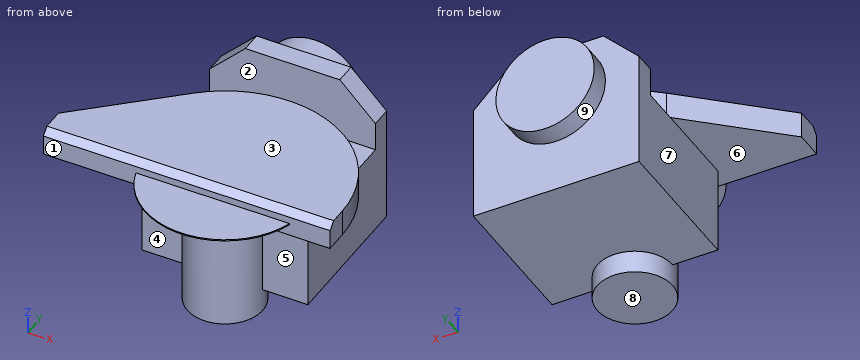
from build123d import *

# Parameters (mm, degrees)
SKETCH1_R                = 225
BOSS_EXTRUDE1_DEPTH      = 3.5
SKETCH2_R                = 105.863842181
BOSS_EXTRUDE2_DEPTH      = 350
SKETCH3_W                = 465.371554394
SKETCH3_H                = 246.036459022
BOSS_EXTRUDE3_DEPTH      = 350
BOSS_EXTRUDE4_DEPTH      = 38
BOSS_EXTRUDE4_DEPTH_BACK = 36
CUT_EXTRUDE1_DEPTH       = 1011
BOSS_EXTRUDE5_DEPTH      = 58
SKETCH7_R                = 138.083103167
BOSS_EXTRUDE6_DEPTH      = 58


with BuildPart() as part:
    # Sketch1 → Boss-Extrude1 (new body)
    with BuildSketch(Plane.XY):
        Circle(SKETCH1_R)
    extrude(amount=BOSS_EXTRUDE1_DEPTH)

    # Sketch2 → Boss-Extrude2 (add)
    with BuildSketch(Plane(origin=(0, 0, 0), x_dir=(-1, 0, 0), z_dir=(0, 0, -1))):
        Circle(SKETCH2_R)
    extrude(amount=BOSS_EXTRUDE2_DEPTH)

    # Sketch3 → Boss-Extrude3 (add)
    with BuildSketch(Plane(origin=(0, 0, 0), x_dir=(1, 0, 0), z_dir=(0, 1, 0))):
        with Locations((0, 162.855088027)):
            Rectangle(SKETCH3_W, SKETCH3_H)
    extrude(amount=BOSS_EXTRUDE3_DEPTH)

    # Sketch4 → Boss-Extrude4 (add, two sides: drawn at the far end of the back side and taken through both)
    with BuildSketch(Plane.XY.offset(3.5).offset(-BOSS_EXTRUDE4_DEPTH_BACK)):
        with BuildLine():
            Line((-475.524623773, -63.931124179), (329.566599898, -63.931124179))
            Line((329.566599898, -63.931124179), (329.566599898, 0))
            ThreePointArc((329.566599898, 0), (133.661871779, 301.245162287), (-221.148477595, 244.351170707))
            Line((-221.148477595, 244.351170707), (-475.524623773, 14.129652631))
            Line((-475.524623773, 14.129652631), (-475.524623773, -63.931124179))
        make_face()
    extrude(amount=BOSS_EXTRUDE4_DEPTH + BOSS_EXTRUDE4_DEPTH_BACK)

    # Sketch5 → Cut-Extrude1 (cut)
    with BuildSketch(Plane(origin=(329.566599898, 0, 0), x_dir=(0, 0, -1), z_dir=(1, 0, 0))):
        Polygon((-41.5, -63.931124179), (-41.5, -45.396753324), (-22.965629146, -63.931124179), align=None)
    extrude(amount=-CUT_EXTRUDE1_DEPTH, mode=Mode.SUBTRACT)

    # Sketch6 → Boss-Extrude5 (add)
    with BuildSketch(Plane(origin=(0, 350, 0), x_dir=(1, 0, 0), z_dir=(0, 1, 0))):
        Polygon((-232.685777197, 285.873317538), (232.685777197, 285.873317538), (232.685777197, -41.230401705), (132.685777197, -141.230401705), (-132.685777197, -141.230401705), (-232.685777197, -41.230401705), align=None)
    extrude(amount=BOSS_EXTRUDE5_DEPTH)

    # Sketch7 → Boss-Extrude6 (add)
    with BuildSketch(Plane(origin=(0, 408, 0), x_dir=(1, 0, 0), z_dir=(0, 1, 0))):
        with Locations(Location((0, 0, 0), (0, 0, 270))):
            Circle(SKETCH7_R)
    extrude(amount=BOSS_EXTRUDE6_DEPTH)


solid = part.part
Can you work these out from the model? Positions are in its coordinate system, mm. Face numbers are marked on the shaded views. A direction names the side the tool comes from. Give positions to 0.01 mm unless a question says otherwise; leave off trailing zeros. Loops run counter-clockwise (first coordinate to the right, second up) from the corner with the lowest first, then second, coordinate; pieces in that order, holes last. Notation, with made-up numbers: (51, -12) - (99, -12) arc R16 cw to (99, 17) - close; hole circle Ø1 at (-34, -14). An arc over 180 degrees is marked (long way). Return JSON: item names as keys, results as strings.
1. For the marked faces 1, 2, 3, 4 and 5, which set-ups out of +Z, -Z, +X, -X, +Y, -Y let a thin tool reach every point of the face, with its end or its side?
Output values:
{"face 1": "-Y", "face 2": "+Z, +X, -X", "face 3": "+Z, +X, -X, -Y", "face 4": "-Z, -X, -Y", "face 5": "-Z, +X, -Y"}
2. I want a section at B-B on z = -275. Please give me the cut outline in (x, y), and give its area (3 significant figures).
Output values:
{"outline": "(-232.69, 0) - (-105.86, 0) arc R105.86 ccw to (105.86, 0) - (232.69, 0) - (232.69, 408) - (-232.69, 408) - close", "area": "207,000 mm²"}
3. I want a section at A-A on x = 0. Please give me the cut outline in (y, z), and give its area (3 significant figures).
Output values:
{"outline": "(-225, 0) - (-105.86, 0) - (-105.86, -350) - (105.86, -350) - (105.86, -285.87) - (408, -285.87) - (408, -138.08) - (466, -138.08) - (466, 138.08) - (408, 138.08) - (408, 141.23) - (350, 141.23) - (350, -39.84) - (105.86, -39.84) - (105.86, -32.5) - (329.57, -32.5) - (329.57, 41.5) - (-45.4, 41.5) - (-63.93, 22.97) - (-63.93, 3.5) - (-225, 3.5) - close", "area": "199,000 mm²"}
4. If I drill on line 1 (Z direction, x = -71, y = 213); line 2 (Z direction, x = -103.5, y = -157); line 3 (Y direction, x = 98, z = -139), over which ranges is the centre line in solid material (lowest first)?
Output values:
{"line 1": "z = -285.87 to -39.84, -32.5 to 41.5", "line 2": "z = 0 to 3.5", "line 3": "y = -40.04 to 408"}
5. I want a section at C-C on y = 133.5. Please give me the cut outline in (x, z).
Output values:
{"outline": "(-343.63, -32.5) - (301.32, -32.5) - (301.32, 41.5) - (-343.63, 41.5) - close; (-232.69, -285.87) - (232.69, -285.87) - (232.69, -39.84) - (-232.69, -39.84) - close"}
6. I'm going to push flat-ended pins straight in: pin 1 Ø1.5 at (x, y) = (175.5, -118.5) entering from +Z; pin 2 Ø3 at (x, y) = (-12, 346) entering from +Z; pin 3 Ø2 at (x, z) = (-229.5, -122.5) entering from +Y. Where does each tip first touch, or does it pass through?
Output values:
{"pin 1": "stops at z = 3.5", "pin 2": "stops at z = -39.84", "pin 3": "stops at y = 408"}
7. I want a section at D-D on y = 56.5. Please give me the cut outline in (x, z).
Output values:
{"outline": "(-428.71, -32.5) - (-89.53, -32.5) - (-89.53, -39.84) - (-232.69, -39.84) - (-232.69, -285.87) - (-89.53, -285.87) - (-89.53, -350) - (89.53, -350) - (89.53, -285.87) - (232.69, -285.87) - (232.69, -39.84) - (89.53, -39.84) - (89.53, -32.5) - (324.69, -32.5) - (324.69, 41.5) - (-428.71, 41.5) - close"}
8. We'd pull the mould along Z, two halves only. Please class the marked faces 6, 7, 8 and 9: +Z half, -Z half, draft (parallel to the pull), parting line (faces both ways), or undercut.
Output values:
{"face 6": "undercut", "face 7": "draft", "face 8": "-Z half", "face 9": "parting line"}
